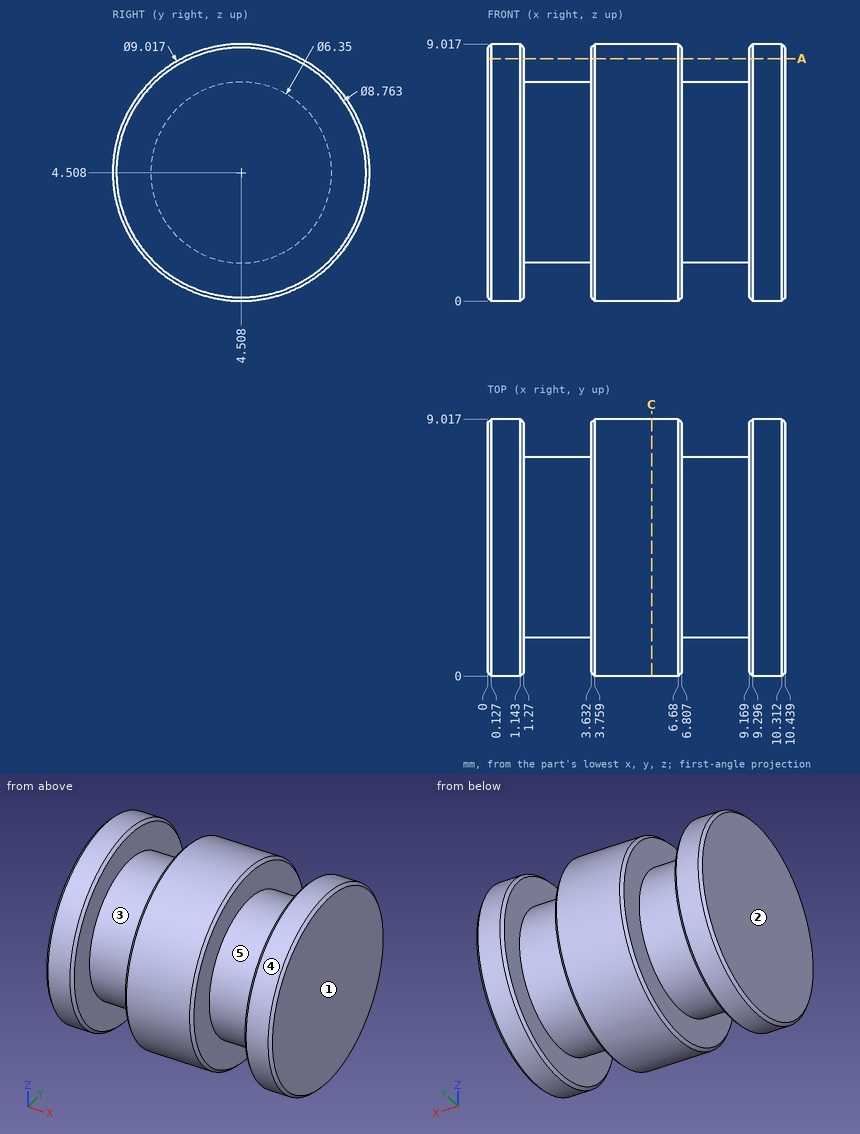
The drawing under review shows one solid part. Ordinate dimensions are in mm from its lowest x, y, z. A direction names the side the tool comes from. Round coordinates to 2 decimals unless told otherwise and drop trailing zeros. Loops run counter-clockwise (first coordinate to the right, second up) from the corner with the lowest first, then second, coordinate; pieces in that order, holes last. Notation, with made-up numbers: (26.5, 44.25) - (37.5, 44.25) arc R21 ccw to (37.5, 74.25) - close; hole circle Ø5 at (72, -10.75). An arc over 180 degrees is marked (long way). One line per question, with ' | ' between items.
Q1. Take a section at A-A (z = 8.5). State how many separate pieces and enclosed holes the cut face has.
Taken from the geometry:
separate pieces: 3 | enclosed holes: 0
Q2. Take a section at C-C (x = 5.75). Give the boundary of the cut face in (y, z).
Taken from the geometry:
outline: circle Ø9.02 at (4.51, 4.51)
Q3. The part is to be moulded in two halves that separate along X. For the marked faces 1, 2 and 3, say which applies: released by +X, released by -X, zero draft, split by the parting line, or undercut.
Taken from the geometry:
face 1: released by +X | face 2: released by -X | face 3: undercut
Q4. For pin 1 (1 mm diameter, centred on x = 1.5, z = 3.5, fed in from -Y); pin 2 (4 mm diameter, centred on x = 8, y = 2.5, fed in from +Z); pin 3 (1.5 mm diameter, centred on x = 8.5, y = 6, fed in from -Z) (1 decimal), all flat-tipped, find the tip position at first contact; note any pin that passes through.
Taken from the geometry:
pin 1: stops at y = 0.05 | pin 2: stops at z = 8.99 | pin 3: stops at z = 0.3
Q5. For line 1 along X through (y, z) = (4.25, 0.5); line 2 along Z through (x, y) = (1, 7.75) (1 decimal); line 3 along Z through (x, y) = (3, 6.75) (1 decimal), list the stretches that pass through material, from the lowest coordinate up. Write a range as [from, to].
Taken from the geometry:
line 1: x = [0, 1.27], [3.63, 6.81], [9.17, 10.44] | line 2: z = [1.4, 7.6] | line 3: z = [2.3, 6.8]
Q6. Tool access review of the marked faces 4 and 5: name each direction out of +Z, -Z, +X, -X, +Y, -Y from which nothing blocks a thin tool from reaching the whole face with its end or side.
Taken from the geometry:
face 4: +X, -X | face 5: none
